Part model, mm, in its own coordinate system. A direction names the side the tool comes from. Round coordinates to 2 decimals unless told otherwise and drop trailing zeros. Loops run counter-clockwise (first coordinate to the right, second up) from the corner with the lowest first, then second, coordinate; pieces in that order, holes last.
from build123d import *

# Parameters (mm, degrees)
BOSS_EXTRUDE1_DEPTH = 250
FILLET1_R           = 5
SKETCH4_R           = 0.75
CUT_EXTRUDE1_DEPTH  = 20
CUT_EXTRUDE2_START  = -20
SKETCH5_R           = 0.75
CUT_EXTRUDE2_DEPTH  = 20


with BuildPart() as part:
    # Sketch1 → Boss-Extrude1 (new body)
    with BuildSketch(Plane.XY):
        Polygon((0, 0), (0, 16), (-3, 16), (-3, 6), (-6.5, 6), (-6.5, 26), (-9.5, 26), (-9.5, 6.5), (-29, 6.5), (-29, 3.5), (-9, 3.5), (-9, 0), (-19, 0), (-19, -3), (0, -3), align=None)
    extrude(amount=BOSS_EXTRUDE1_DEPTH)

    # Fillet1
    # the kernel refuses this fillet: 5 mm, written as the material it adds along each edge
    with BuildSketch(Plane(origin=(-9.5, 6.5, 0), x_dir=(-1, 0, 0), z_dir=(0, 0, 1))) as fillet1_piece_1:
        with BuildLine():
            CenterArc((FILLET1_R, -FILLET1_R), FILLET1_R, 90, 90)
            Line((0, -FILLET1_R), (0, 0))
            Line((0, 0), (FILLET1_R, 0))
        make_face()
    extrude(amount=250)
    # the kernel refuses this fillet: 5 mm, written as the material it takes off along each edge
    with BuildSketch(Plane(origin=(-19, -3, -11.456439237), x_dir=(1, 0, 0), z_dir=(0, 0, 1))) as fillet1_2_piece_1:
        with BuildLine():
            CenterArc((4.582575695, 5), FILLET1_R, 203.578178478, 66.421821522)
            Line((0, 3), (0, 0))
            Line((0, 0), (4.582575695, 0))
        make_face()
    extrude(amount=272.912878475, mode=Mode.SUBTRACT)
    with BuildSketch(Plane(origin=(0, -3, -12.5), x_dir=(0, 1, 0), z_dir=(0, 0, 1))) as fillet1_2_piece_2:
        with BuildLine():
            CenterArc((FILLET1_R, FILLET1_R), FILLET1_R, 180, 90)
            Line((0, FILLET1_R), (0, 0))
            Line((0, 0), (FILLET1_R, 0))
        make_face()
    extrude(amount=275, mode=Mode.SUBTRACT)
    with BuildSketch(Plane(origin=(0, 16, -11.456439237), x_dir=(0, -1, 0), z_dir=(0, 0, 1))) as fillet1_2_piece_3:
        with BuildLine():
            CenterArc((4.582575695, -5), FILLET1_R, 90, 66.421821522)
            Line((0, -3), (0, 0))
            Line((0, 0), (4.582575695, 0))
        make_face()
    extrude(amount=272.912878475, mode=Mode.SUBTRACT)

    # Sketch4 → Cut-Extrude1 (cut)
    with BuildSketch(Plane(origin=(0, 0, 0), x_dir=(-1, 0, 0), z_dir=(0, 0, -1))):
        with Locations((4.75, 1.75)):
            Circle(SKETCH4_R)
    extrude(amount=-CUT_EXTRUDE1_DEPTH, mode=Mode.SUBTRACT)

    # Sketch5 → Cut-Extrude2 (cut)
    with BuildSketch(Plane.XY.offset(250).offset(CUT_EXTRUDE2_START)):
        with Locations(Location((-4.75, 1.75, 0), (0, 0, 180))):
            Circle(SKETCH5_R)
    extrude(amount=CUT_EXTRUDE2_DEPTH, mode=Mode.SUBTRACT)


solid = part.part
1) Drop flat-ended pins along their axis: pin 1 Ø4 at (x, z) = (-5.5, 130) entering from +Y; pin 2 Ø10 at (x, z) = (-20, 67) entering from -Y; pin 3 Ø1.5 at (y, z) = (15.5, 63) entering from -X; pin 4 Ø11 at (x, z) = (-15.5, 167) entering from +Y. Give the stop position or say it passes through.
Values:
pin 1: stops at y = 26
pin 2: stops at y = -2.97
pin 3: stops at x = -9.5
pin 4: stops at y = 9.32
2) Slice it at B-B, the plane z = 227. Give the cut face in (x, y).
Values:
outline: (-29, 3.5) - (-9, 3.5) - (-9, 0) - (-19, 0) arc R5 ccw to (-14.42, -3) - (-5, -3) arc R5 ccw to (0, 2) - (0, 11.42) arc R5 ccw to (-3, 16) - (-3, 6) - (-6.5, 6) - (-6.5, 26) - (-9.5, 26) - (-9.5, 11.5) arc R5 cw to (-14.5, 6.5) - (-29, 6.5) - close
3) Slice it at C-C, the plane y = 22.75. Give the cut face in (x, z), then the cut area to 3 significant figures.
Values:
outline: (-9.5, 0) - (-6.5, 0) - (-6.5, 250) - (-9.5, 250) - close
area: 750 mm2
4) Slice it at D-D, the plane x = -24. Give the cut face in (y, z).
Values:
outline: (3.5, 0) - (6.5, 0) - (6.5, 250) - (3.5, 250) - close
5) Mould opens along X. For faces 6 (the face through (-22, 6.5, 123)), 7 (the face through (-0.795, 14.122, 123.25)), 8 (the face through (-6.5, 16, 123)) say: released by +X, released by -X, zero draft, split by the parting line, or undercut.
Values:
face 6: zero draft
face 7: released by +X
face 8: undercut
6) Slice it at A-A, the plane y = 8.75. Give the cut face in (x, z), then the cut area to 3 significant figures.
Values:
outline: (-10.32, 0) - (-6.5, 0) - (-6.5, 250) - (-10.32, 250) - close; (-3, 0) - (0, 0) - (0, 250) - (-3, 250) - close
area: 1,710 mm2
7) Tool access for faces 1 (the face through (-3, 11, 123)), 2 (the face through (-14, 0, 123)), 3 (the face through (-9.5, 19, 123)), 4 (the face through (-2, -2, 123)), 5 (the face through (-9, 7, 250)): list every direction of +Z, -Z, +X, -X, +Y, -Y with a clear straight run to the whole face (end or side of a thin tool).
Values:
face 1: +Z, -Z, +Y
face 2: +Z, -Z, -X
face 3: +Z, -Z, -X, +Y
face 4: +Z, -Z, +X, -Y
face 5: +Z, +X, -X, +Y, -Y
8) Wall check: line 1 along Y through (x, z) = (-4.75, 241); line 2 along X through (y, z) = (1.75, 235.25); line 3 along X through (y, z) = (22.25, 237). Give the ranges that are in metal, low to high.
Values:
line 1: y = -2.99 to 1, 2.5 to 6
line 2: x = -9 to -5.5, -4 to -0.01
line 3: x = -9.5 to -6.5
